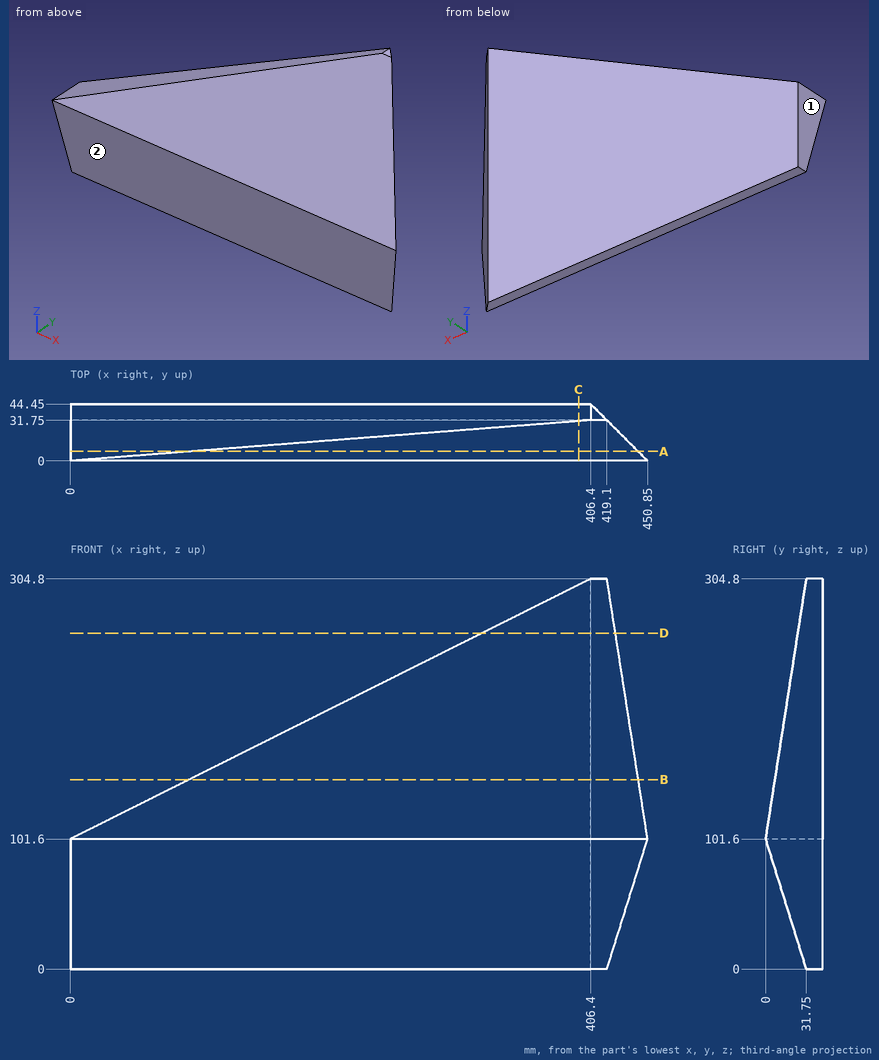
The drawing under review shows one solid part. Ordinate dimensions are in mm from its lowest x, y, z. Give positions to 0.01 mm unless a question says otherwise; leave off trailing zeros. Write each loop counter-clockwise with the first axis right and the second up, starting at its lowest first coordinate (ties: lowest second). Pieces come first, ordered by that corner, then holes. Notation, with made-up numbers: M 77,-2.5 L 128,-2.5 A29 ccw 128,20.5 Z; hole C 27.25,71.25 d2. An arc over 180 degrees is marked long. Write each question's results on one line, items separated by ' | '. Start each with the question number.
1. Mouldability with a two-part tool opening along X and no side actions: class the marked faces 1 and 2 as released by +X, released by -X, zero draft, split by the parting line, or undercut.
2. Insertion check: pin 1 Ø1 at (x, y) = (309.5, 32) entering from +Z; pin 2 Ø1.5 at (y, z) = (30.5, 208.5) entering from +X; pin 3 Ø10 at (x, y) = (174.5, 33) entering from +Z. Each pin has a flat end and moves straight along its axis. Give the tip position at first contact, or say it passes through.
3. We need section C-C (x = 397). Write out the cut boundary in (y, z), and give its area (3 significant figures).
4. We need section D-D (z = 262.5). Write out the cut boundary in (x, y).
5. We need section A-A (y = 7.5). Write out the cut boundary in (x, z).
6. For probe 1 along Z at (x, y) = (326.5, 34); probe 2 along Y at (x, z) = (366, 220.5); probe 3 along Y at (x, z) = (322, 108), list the stretches that pass through material, from the lowest coordinate up. Write a range as [from, to].
7. We need section B-B (z = 148). Write out the cut boundary in (x, y), and give its area (3 significant figures).
Results found:
1) face 1: released by -X | face 2: zero draft
2) pin 1: stops at z = 256.6 | pin 2: stops at x = 421.1 | pin 3: stops at z = 191.35
3) outline: M 0,101.6 L 31.75,0 L 44.45,0 L 44.45,300.1 L 31.02,300.1 Z | area: 8,650 mm^2
4) outline: M 321.8,25.14 L 425.71,25.14 L 406.4,44.45 L 321.8,44.45 Z
5) outline: M 0,77.6 L 443.35,77.6 L 443.35,149.6 L 96,149.6 L 0,101.6 Z
6) probe 1: z = [0, 264.85] | probe 2: y = [18.58, 44.45] | probe 3: y = [1, 44.45]
7) outline: M 92.8,7.25 L 443.6,7.25 L 406.4,44.45 L 92.8,44.45 Z | area: 12,400 mm^2
